from build123d import *

# Parameters (mm, degrees)
SKETCH_1_W                   = 21.25
SKETCH_1_H                   = 4
HOLE_WIZARD_M6_1_D           = 6.6
HOLE_WIZARD_M6_1_CBORE_D     = 11
HOLE_WIZARD_M6_1_CBORE_DEPTH = 0.5


with BuildPart() as part:
    # 草图1 → 旋转1 (revolve)
    with BuildSketch(Plane.XY, mode=Mode.PRIVATE) as revolve_1_sk:
        with Locations((19.375, 2)):
            Rectangle(SKETCH_1_W, SKETCH_1_H)
    revolve(revolve_1_sk.sketch.rotate(Axis((0, 4, 0), (0, -1, 0)), 180), axis=Axis((0, 4, 0), (0, -1, 0)))

    # M6 六角头螺栓的柱形沉头孔1 (through all)
    with Locations(Plane(origin=(0, 4, 0), x_dir=(1, 0, 0), z_dir=(0, 1, 0))):
        with Locations((15, 0), (0, -15), (-15, 0), (0, 15)):
            CounterBoreHole(HOLE_WIZARD_M6_1_D / 2, HOLE_WIZARD_M6_1_CBORE_D / 2, HOLE_WIZARD_M6_1_CBORE_DEPTH)


solid = part.part
Design review of the part built by this model. Coordinates are the model's own, in mm. A direction names the side the tool comes from. Give positions to 0.01 mm unless a question says otherwise; leave off trailing zeros. Write each loop counter-clockwise with the first axis right and the second up, starting at its lowest first coordinate (ties: lowest second). Pieces come first, ordered by that corner, then holes. Notation, with made-up numbers: M 44.5,70.25 L 94.5,70.25 A11 cw 94.5,86.25 Z; hole C 70.25,78.5 d7. An arc over 180 degrees is marked long. Answer as a JSON object with one key per item and string values. Group by question number.
1) We need section C-C (z = 1). Give the boundary of the cut face in (x, y).
2) Clearance check with a flat-ended pin moving along its axis: pin 1 Ø7.5 at (x, z) = (-15, 0) entering from +Y. State where the tip first meets the part, or that it passes through.
3) Mouldability with a two-part tool opening along Z and no side actions: class faces 3 (the face through (-16.128, 2.028, -25.296)), 4 (the face through (6, 0, -7)), 5 (the face through (1.9, 2.03, 8.54)) as released by +Z, released by -Z, zero draft, split by the parting line, or undercut.
4) Tool access review of faces 1 (the face through (-15, 3.5, 4)), 2 (the face through (2.43, 1.73, -17.23)): name each direction out of +Z, -Z, +X, -X, +Y, -Y from which nothing blocks a thin tool from reaching the whole face with its end or side.
5) We need section A-A (x = 0). Give the boundary of the cut face in (y, z), and give its area (3 significant figures).
6) We need section B-B (z = 15). Give the boundary of the cut face in (x, y), and give its area (3 significant figures).
7) For line 1 along Z through (x, y) = (0, 3.95); line 2 along Z through (x, y) = (0, 0.8); line 3 along X through (y, z) = (0.25, 1.5), list the stretches that pass through material, from the lowest coordinate up.
8) We need section D-D (y = 1.4). Give the boundary of the cut face in (x, z), and give its area (3 significant figures).
Answer key:
{
 "1": {"outline": "M -29.98,0 L -18.14,0 L -18.14,3.5 L -20.41,3.5 L -20.41,4 L -29.98,4 Z; M -11.86,0 L -8.69,0 L -8.69,4 L -9.59,4 L -9.59,3.5 L -11.86,3.5 Z; M 8.69,0 L 11.86,0 L 11.86,3.5 L 9.59,3.5 L 9.59,4 L 8.69,4 Z; M 18.14,0 L 29.98,0 L 29.98,4 L 20.41,4 L 20.41,3.5 L 18.14,3.5 Z"},
 "2": {"pin 1": "stops at y = 3.5"},
 "3": {"face 3": "split by the parting line", "face 4": "zero draft", "face 5": "undercut"},
 "4": {"face 1": "+Y", "face 2": "+Y, -Y"},
 "5": {"outline": "M 0,-30 L 4,-30 L 4,-20.5 L 3.5,-20.5 L 3.5,-18.3 L 0,-18.3 Z; M 0,-11.7 L 3.5,-11.7 L 3.5,-9.5 L 4,-9.5 L 4,-8.75 L 0,-8.75 Z; M 0,8.75 L 4,8.75 L 4,9.5 L 3.5,9.5 L 3.5,11.7 L 0,11.7 Z; M 0,18.3 L 3.5,18.3 L 3.5,20.5 L 4,20.5 L 4,30 L 0,30 Z", "area": "113 mm²"},
 "6": {"outline": "M -25.98,0 L -3.3,0 L -3.3,3.5 L -5.5,3.5 L -5.5,4 L -25.98,4 Z; M 3.3,0 L 25.98,0 L 25.98,4 L 5.5,4 L 5.5,3.5 L 3.3,3.5 Z", "area": "179 mm²"},
 "7": {"line 1": "z = -30 to -20.5, -9.5 to -8.75, 8.75 to 9.5, 20.5 to 30", "line 2": "z = -30 to -18.3, -11.7 to -8.75, 8.75 to 11.7, 18.3 to 30", "line 3": "x = -29.96 to -17.94, -12.06 to -8.62, 8.62 to 12.06, 17.94 to 29.96"},
 "8": {"outline": "C 0,0 d60; hole C -15,0 d6.6; hole C 0,0 d17.5; hole C 0,-15 d6.6; hole C 0,15 d6.6; hole C 15,0 d6.6", "area": "2,450 mm²"}
}
